Design review of the part built by this model. Coordinates are the model's own, in mm. Face numbers are marked on the shaded views. Coordinates: 2 decimals unless noted, no trailing zeros. Write each loop counter-clockwise with the first axis right and the second up, starting at its lowest first coordinate (ties: lowest second). Pieces come first, ordered by that corner, then holes.
Q1. Add section A-A, the plane x = -1.25. Give the boundary of the cut face in (y, z), plus the area to 3 significant figures.
Q2. The part is to be moulded in two halves that separate along X. For the marked faces 1, 2 and 3, say which applies: +X half, -X half, draft (parallel to the pull), parting line (faces both ways), or undercut.
Q3. To check wall thickness, follow probe 1 along X at (y, z) = (2.1, -8); probe 2 along X at (y, z) = (2.4, -7); probe 3 along Z at (x, y) = (0.25, 2.2). State the ranges of each line that lie inside material, in increasing order.
Q4. Clearance check with flat-ended pins moving along their axes: pin 1 Ø0.6 at (y, z) = (2, -10) entering from -X; pin 2 Ø1 at (y, z) = (1.5, -11.5) entering from +X; pin 3 Ø1 at (y, z) = (1, -28) entering from -X. State where each tip first meets the part, or that it passes through.
Q5. Add section C-C, the plane z = -3.5. Give the boundary of the cut face in (x, y), plus the area to 3 significant figures.
Q6. Add section B-B, the plane y = 1.7. Give the boundary of the cut face in (x, z), plus the area to 3 significant figures.
from build123d import *

# Parameters (mm, degrees)
BOSS_EXTRUDE1_DEPTH = 33
SKETCH2_W           = 7
SKETCH2_H           = 7
CUT_EXTRUDE1_DEPTH  = 2
FILLET1_R           = 13


with BuildPart() as part:
    # Sketch1 → Boss-Extrude1 (new body)
    with BuildSketch(Plane.XY):
        Polygon((-12.134314575, 2.8), (-14.534314575, 0.4), (14.534314575, 0.4), (12.134314575, 2.8), align=None)
    extrude(amount=-BOSS_EXTRUDE1_DEPTH)

    # Sketch2 → Cut-Extrude1 (cut)
    with BuildSketch(Plane(origin=(0, 2.8, 0), x_dir=(1, 0, 0), z_dir=(0, 1, 0))):
        with Locations((0, 8.5)):
            Rectangle(SKETCH2_W, SKETCH2_H)
    extrude(amount=-CUT_EXTRUDE1_DEPTH, mode=Mode.SUBTRACT)

    # Fillet1
    # the kernel refuses this fillet: 13 mm, written as the material it adds along each edge
    with BuildSketch(Plane(origin=(-3.5, 0.8, -12), x_dir=(0, 1, 0), z_dir=(1, 0, 0))) as fillet1_piece_1:
        with BuildLine():
            CenterArc((13, 6.92820323), FILLET1_R, 180, 32.204227504)
            Line((0, 6.92820323), (0, 0))
            Line((0, 0), (2, 0))
        make_face()
    extrude(amount=7)


solid = part.part
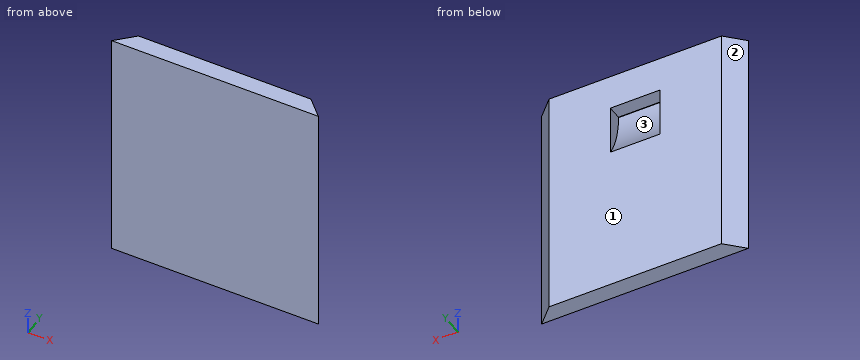
Here are the results:
1. outline: (0.4, -33) - (2.8, -33) - (2.8, -12) arc R13 cw to (0.8, -5.07) - (0.8, -5) - (2.8, -5) - (2.8, 0) - (0.4, 0) - close
1. area: 69.7 mm2
2. face 1: draft
2. face 2: -X half
2. face 3: undercut
3. probe 1: x = -12.83 to -3.5, 3.5 to 12.83
3. probe 2: x = -12.53 to -3.5, 3.5 to 12.53
3. probe 3: z = -33 to -10.94, -5 to 0
4. pin 1: stops at x = -13.23
4. pin 2: stops at x = 13.93
4. pin 3: stops at x = -14.43
5. outline: (-14.53, 0.4) - (14.53, 0.4) - (12.13, 2.8) - (-12.13, 2.8) - close
5. area: 64.0 mm2
6. outline: (-13.23, -33) - (13.23, -33) - (13.23, 0) - (-13.23, 0) - close; hole (-3.5, -9.82) - (3.5, -9.82) - (3.5, -5) - (-3.5, -5) - close
6. area: 840 mm2
